from build123d import *

# Parameters (mm, degrees)
F1_DEPTH = 12.7
F2_R     = 4.7625
F3_DEPTH = 12.701
F4_W     = 203.2
F4_H     = 9.79558
F5_DEPTH = 12.701
F7_DEPTH = 12.701


with BuildPart() as f1:
    # F0 (on Top) → F1 (new body)
    with BuildSketch(Plane.XY):
        with BuildLine():
            Line((208.057067, 25.4), (-305.252269, 25.4))
            ThreePointArc((-305.252269, 25.4), (-318.722653, 19.820384), (-324.302269, 6.35))
            Line((-324.302269, 6.35), (-324.302269, -82.55))
            ThreePointArc((-324.302269, -82.55), (-318.722653, -96.020384), (-305.252269, -101.6))
            Line((-305.252269, -101.6), (469.447731, -101.6))
            ThreePointArc((469.447731, -101.6), (482.918115, -96.020384), (488.497731, -82.55))
            Line((488.497731, -82.55), (488.497731, 6.35))
            ThreePointArc((488.497731, 6.35), (482.918115, 19.820384), (469.447731, 25.4))
            Line((469.447731, 25.4), (464.684607, 25.4))
            ThreePointArc((464.684607, 25.4), (463.109975, 25.302005), (461.559644, 25.009533))
            Line((461.559644, 25.009533), (365.61775, 0.653221))
            ThreePointArc((365.61775, 0.653221), (363.032974, 0.274247), (360.425341, 0.432165))
            Line((360.425341, 0.432165), (210.124513, 25.230589))
            ThreePointArc((210.124513, 25.230589), (209.094255, 25.357576), (208.057067, 25.4))
        make_face()
    extrude(amount=F1_DEPTH)

    # F2 (on face) → F3 (cut, through all)
    with BuildSketch(Plane.XY.offset(12.7)):
        with Locations((-286.202269, 0)):
            Circle(F2_R)
        with Locations((-286.202269, -50.8)):
            Circle(F2_R)
        with Locations((-210.002269, 0)):
            Circle(F2_R)
        with Locations((450.397731, 0)):
            Circle(F2_R)
        with Locations((450.397731, -50.8)):
            Circle(F2_R)
    extrude(amount=-F3_DEPTH, mode=Mode.SUBTRACT)

    # F4 (on face) → F5 (cut, through all)
    with BuildSketch(Plane.XY.offset(12.7)):
        with Locations((310.697731, -71.30221)):
            Rectangle(F4_W, F4_H)
        with Locations((310.697731, -45.90221)):
            Rectangle(F4_W, F4_H)
        with Locations((82.097731, -45.90221)):
            Rectangle(F4_W, F4_H)
        with Locations((82.097731, -71.30221)):
            Rectangle(F4_W, F4_H)
        with Locations((-146.502269, -71.30221)):
            Rectangle(F4_W, F4_H)
        with Locations((-146.502269, -45.90221)):
            Rectangle(F4_W, F4_H)
    extrude(amount=-F5_DEPTH, mode=Mode.SUBTRACT)

    # F6 (on face) → F7 (cut, through all)
    with BuildSketch(Plane.XY.offset(12.7)):
        Polygon((-137.433179, -19.05), (-181.427269, 6.35), (-184.602269, 0.850739), (-140.608179, -24.549261), align=None)
        Polygon((-86.633179, -19.05), (-130.627269, 6.35), (-133.802269, 0.850739), (-89.808179, -24.549261), align=None)
        Polygon((-35.833179, -19.05), (-79.827269, 6.35), (-83.002269, 0.850739), (-39.008179, -24.549261), align=None)
        Polygon((14.966821, -19.05), (-29.027269, 6.35), (-32.202269, 0.850739), (11.791821, -24.549261), align=None)
        Polygon((65.766821, -19.05), (21.772731, 6.35), (18.597731, 0.850739), (62.591821, -24.549261), align=None)
        Polygon((116.566821, -19.05), (72.572731, 6.35), (69.397731, 0.850739), (113.391821, -24.549261), align=None)
        Polygon((167.366821, -19.05), (123.372731, 6.35), (120.197731, 0.850739), (164.191821, -24.549261), align=None)
        Polygon((218.166821, -19.05), (174.172731, 6.35), (170.997731, 0.850739), (214.991821, -24.549261), align=None)
    extrude(amount=-F7_DEPTH, mode=Mode.SUBTRACT)


solid = f1.part
The listing builds one solid part. Answer for the finished solid, in the listing's coordinates (mm). A direction names the side the tool comes from. Round coordinates to 2 decimals unless told otherwise and drop trailing zeros. Write each loop counter-clockwise with the first axis right and the second up, starting at its lowest first coordinate (ties: lowest second). Pieces come first, ordered by that corner, then holes. Notation, with made-up numbers: M 34,-24 L 49,-24 A23 cw 49,-8 Z; hole C 33,38.25 d1. An arc over 180 degrees is marked long. Write each question's results on one line, items separated by ' | '. Start each with the question number.
Item 1: Straight lines are drawn through the part: probe 1 along X at (y, z) = (-71, 1); probe 2 along Y at (x, z) = (357, 7.5); probe 3 along Y at (x, z) = (44, 2.75). For each, find the intervals that lie inside material, in ascending order.
Item 2: Find section C-C on z = 2.25. Give the number of separate pieces and of enclosed holes in the cut face, and give its area (3 significant figures).
Item 3: The mould has two halves that part along Y. Classify faces 1 (the flat face through (309, -41.004, 6)), 2 (the flat face through (94.88, -6.53, 6.44)), 3 (the flat face through (77, -101.6, 6)), 4 (the flat face through (488.498, -39, 6)): +Y half, -Y half, draft (parallel to the pull), parting line (faces both ways), or undercut.
Item 4: Find section B-B on x = 137.5. Write down the section's boundary in (y, z), and give its area (3 significant figures).
Item 5: Find section A-A on x = 383. Write down the section's boundary in (y, z), and give its area (3 significant figures).
Item 6: Given pin 1 Ø2 at (x, y) = (206, -2.5) entering from -Z, flat-ended and moving along its own axis, determine where the tip first touches the part or whether it passes through.
Item 7: Which of the six approach directions +Z, -Z, +X, -X, +Y, -Y give full straight-line access (tool end or side, diameter ignored) to faces 5 (the flat face through (-45, 25.4, 6)), 6 (the flat face through (-159.12, -6.53, 6.44))?
Answer block:
1) probe 1: x = -324.3 to -248.1, -44.9 to -19.5, 183.7 to 209.1, 412.3 to 488.5 | probe 2: y = -101.6 to -76.2, -66.4 to -50.8, -41 to 1 | probe 3: y = -101.6 to -76.2, -66.4 to -50.8, -41 to -13.82, -6.48 to 25.4
2) separate pieces: 1 | enclosed holes: 19 | area: 84,800 mm²
3) face 1: undercut | face 2: undercut | face 3: -Y half | face 4: draft
4) outline: M -101.6,0 L -76.2,0 L -76.2,12.7 L -101.6,12.7 Z; M -66.4,0 L -50.8,0 L -50.8,12.7 L -66.4,12.7 Z; M -41,0 L -9.14,0 L -9.14,12.7 L -41,12.7 Z; M -1.81,0 L 25.4,0 L 25.4,12.7 L -1.81,12.7 Z | area: 1,270 mm²
5) outline: M -101.6,0 L -76.2,0 L -76.2,12.7 L -101.6,12.7 Z; M -66.4,0 L -50.8,0 L -50.8,12.7 L -66.4,12.7 Z; M -41,0 L 5.07,0 L 5.07,12.7 L -41,12.7 Z | area: 1,110 mm²
6) pin 1: stops at z = 0
7) face 5: +Z, -Z, +X, -X, +Y | face 6: +Z, -Z
